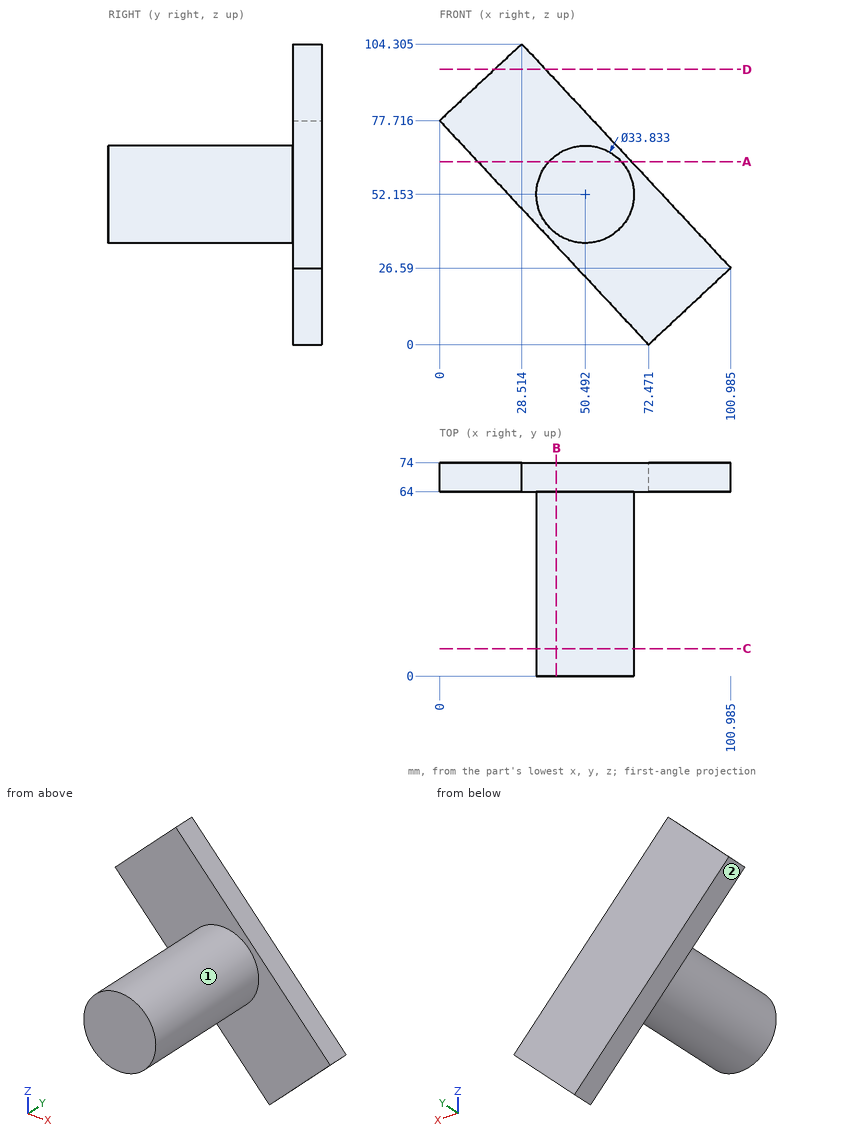
Verification items for this drawing (mm, ordinates from the low corner). A direction names the side the tool comes from. Round coordinates to 2 decimals unless told otherwise and drop trailing zeros. Loops run counter-clockwise (first coordinate to the right, second up) from the corner with the lowest first, then second, coordinate; pieces in that order, holes last. Notation, with made-up numbers: (37.25, 27.5) - (75.25, 27.5) arc R26 ccw to (75.25, 46.5) - close; hole circle Ø1 at (88.5, -19). An arc over 180 degrees is marked (long way). Write item = value, one per line.
Q1. Material ranges on L1, parallel to Y at x = 61, z = 33; L2, parallel to Z at x = 50.5, y = 21; L3, parallel to Z at x = 40, y = 71 (1 decimal), recorded low to high.
Here are the results:
L1 = 64 to 74
L2 = 35.24 to 69.07
L3 = 34.8 to 92
Q2. Sectioned sample at C-C on y = 9.5. Record the boundary of the cut face in (x, z), plus the area to 3 significant figures.
Here are the results:
outline = circle Ø33.83 at (50.49, 52.15)
area = 899 mm^2
Q3. Depth check by flat-ended pin: pin 1 (1.5 mm diameter, centred on x = 35, z = 58, fed in from -Y); pin 2 (1.5 mm diameter, centred on x = 11, z = 85, fed in from -Y); pin 3 (10 mm diameter, centred on y = 60.5, z = 36.5, fed in from -X) (1 decimal); pin 4 (8 mm diameter, centred on x = 65.5, y = 26, fed in from -Z). Enter the tip coordinate at first touch or a pass-through.
Here are the results:
pin_1 = 0
pin_2 = 64
pin_3 = 35.1
pin_4 = 39.31
Q4. Sectioned sample at B-B on x = 40.5. Record the boundary of the cut face in (y, z) (1 decimal), plus the area to 3 significant figures.
Here are the results:
outline = (0, 38.5) - (64, 38.5) - (64, 34.3) - (74, 34.3) - (74, 91.5) - (64, 91.5) - (64, 65.8) - (0, 65.8) - close
area = 2,320 mm^2
Q5. Sectioned sample at A-A on z = 63.5. Record the boundary of the cut face in (x, y) (1 decimal).
Here are the results:
outline = (13.3, 64) - (37.9, 64) - (37.9, 0) - (63, 0) - (63, 64) - (66.6, 64) - (66.6, 74) - (13.3, 74) - close
Q6. Sectioned sample at D-D on z = 95.5. Record the boundary of the cut face in (x, y) (1 decimal).
Here are the results:
outline = (19.1, 64) - (36.7, 64) - (36.7, 74) - (19.1, 74) - close
Q7. Tool access check on the marked faces 1 and 2. Record the directions out of +Z, -Z, +X, -X, +Y, -Y that give a thin tool (end or side, any length) a straight path to the whole face; none if there is none.
Here are the results:
face_1 = -Y
face_2 = -Z, -X, +Y, -Y
